Can you work these out from the model? Positions are in its coordinate system, mm. Face numbers are marked on the shaded views. A direction names the side the tool comes from. Give positions to 0.01 mm unless a question says otherwise; leave off trailing zeros. Write each loop counter-clockwise with the first axis right and the second up, starting at its lowest first coordinate (ties: lowest second). Pieces come first, ordered by that corner, then holes.
1. Thinking about a two-plate mould opening in Z: for the marked faces 1, 2, 3 and 4, which applies, pulls with the +Z half, pulls with the -Z half, needs draft (parallel to the pull), parting line crosses it, or undercut?
2. Suppose I cut it at B-B (y = -18). Please give me the cut outline in (x, z), and give its area (3 significant figures).
3. Suppose I cut it at A-A (x = 20). Please give me the cut outline in (y, z), and give its area (3 significant figures).
4. On a 3-axis mill with a long thin cutter (end or side, diameter ignored), from which of +Z, -Z, +X, -X, +Y, -Y can I reach the whole of each face in a straight line? I mean the marked faces 5, 6 and 7. Say none if no direction works.
5. Suppose I cut it at C-C (z = -28). Please give me the cut outline in (x, y).
6. If I drill on probe 1 along Y at (x, z) = (20, 3.85); probe 2 along X at (y, z) = (-18, 1.2); probe 3 along Y at (x, z) = (-37, -26.55), over which ranges is the centre line in solid material (lowest first)?
7. I'm going to push flat-ended pins straight in: pin 1 (1 mm diameter, centred on y = -2, z = -10.5, fed in from +X); pin 2 (10.5 mm diameter, centred on y = -10, z = -16, fed in from -X); pin 3 (3 mm diameter, centred on y = -10, z = -17, fed in from +X); pin 4 (4 mm diameter, centred on x = -21, y = -18.5, fed in from +Z). Where does each tip first touch, or does it pass through?
8. Suppose I cut it at D-D (y = 18). Please give me the cut outline in (x, z), and give its area (3 significant figures).
```python
from build123d import *

# Parameters (mm, degrees)
SKETCH1_W                      = 60
SKETCH1_H                      = 50
BOSS_EXTRUDE1_DEPTH            = 5
CUT_EXTRUDE1_DEPTH             = 40.37003937
CUT_EXTRUDE1_DEPTH_BACK        = 40.37003937
SKETCH5_R                      = 1.75
BOSS_EXTRUDE2_START            = -17
BOSS_EXTRUDE2_DEPTH            = 35
SKETCH6_W                      = 5.5
SKETCH6_H                      = 50
BOSS_EXTRUDE3_DEPTH            = 33
CUT_EXTRUDE2_DEPTH             = 71.32780389
CUT_EXTRUDE2_DEPTH_BACK        = 71.32780389
SKETCH7_R                      = 1.75
FILLET2_R                      = 3
FILLET3_R                      = 3
SKETCH8_R                      = 10.5
CUT_EXTRUDE3_DEPTH             = 28
FILLET4_R                      = 5
CBORE_FOR_M3_SHCS1_D           = 3.4
CBORE_FOR_M3_SHCS1_CBORE_D     = 6.5
CBORE_FOR_M3_SHCS1_CBORE_DEPTH = 3
SKETCH16_R                     = 1.7
CUT_EXTRUDE4_DEPTH             = 3
CHAMFER1_SIZE                  = 4


with BuildPart() as part:
    # Sketch1 → Boss-Extrude1 (new body)
    with BuildSketch(Plane.XY):
        Rectangle(SKETCH1_W, SKETCH1_H)
    extrude(amount=BOSS_EXTRUDE1_DEPTH)

    # Sketch5 → Cut-Extrude1 (cut, two sides: drawn at the far end of the back side and taken through both)
    with BuildSketch(Plane.XY.offset(5).offset(-CUT_EXTRUDE1_DEPTH_BACK)):
        with Locations((-20, 18)):
            Circle(SKETCH5_R)
        with Locations((20, 18)):
            Circle(SKETCH5_R)
        with Locations((20, -18)):
            Circle(SKETCH5_R)
        with Locations((-20, -18)):
            Circle(SKETCH5_R)
    extrude(amount=CUT_EXTRUDE1_DEPTH + CUT_EXTRUDE1_DEPTH_BACK, mode=Mode.SUBTRACT)

    # Sketch2 → Boss-Extrude2 (add)
    with BuildSketch(Plane(origin=(30, 0, 0), x_dir=(0, 0, -1), z_dir=(1, 0, 0)).offset(BOSS_EXTRUDE2_START)):
        Polygon((0, -25), (31, -25), (31, 25), (25.5, 25), (25.5, 8), (5.5, 8), (5.5, 25), (0, 25), align=None)
    extrude(amount=-BOSS_EXTRUDE2_DEPTH)

    # Sketch6 → Boss-Extrude3 (add)
    with BuildSketch(Plane.ZY.offset(22)):
        with Locations((-28.25, 0)):
            Rectangle(SKETCH6_W, SKETCH6_H)
    extrude(amount=BOSS_EXTRUDE3_DEPTH)

    # Sketch7 → Cut-Extrude2 (cut, two sides: drawn at the far end of the back side and taken through both)
    with BuildSketch(Plane(origin=(0, 0, -31), x_dir=(-1, 0, 0), z_dir=(0, 0, -1)).offset(-CUT_EXTRUDE2_DEPTH_BACK)):
        with Locations((37, 7.5)):
            Circle(SKETCH7_R)
        with Locations((44.5, 0)):
            Circle(SKETCH7_R)
        with Locations((37, -7.5)):
            Circle(SKETCH7_R)
        with Locations((29.5, 0)):
            Circle(SKETCH7_R)
    extrude(amount=CUT_EXTRUDE2_DEPTH + CUT_EXTRUDE2_DEPTH_BACK, mode=Mode.SUBTRACT)

    # Fillet2
    fillet2_edges = [part.edges().sort_by_distance(p)[0] for p in [
        (-22, 0, 0),
        (13, 0, 0),
    ]]
    fillet(fillet2_edges, radius=FILLET2_R)

    # Fillet3
    fillet3_edges = [part.edges().sort_by_distance(p)[0] for p in [
        (-4.5, 8, -5.5),
        (-4.5, 8, -25.5),
    ]]
    fillet(fillet3_edges, radius=FILLET3_R)

    # Sketch8 → Cut-Extrude3 (cut)
    with BuildSketch(Plane(origin=(0, 0, -31), x_dir=(-1, 0, 0), z_dir=(0, 0, -1))):
        with Locations((5, -10)):
            Circle(SKETCH8_R)
        with BuildLine():
            Line((-5.5, 0.5), (-5.5, -10))
            ThreePointArc((-5.5, -10), (-2.424621218, -2.575378813), (4.999999956, 0.5))
            Line((4.999999956, 0.5), (-5.5, 0.5))
        make_face()
        with BuildLine():
            ThreePointArc((4.999999956, 0.5), (12.424621187, -2.575378782), (15.5, -10))
            Line((15.5, -10), (15.5, 0.5))
            Line((15.5, 0.5), (4.999999956, 0.5))
        make_face()
        with BuildLine():
            Line((-5.5, -10), (-5.5, -20.5))
            Line((-5.5, -20.5), (5, -20.5))
            ThreePointArc((5, -20.5), (-2.424621202, -17.424621202), (-5.5, -10))
        make_face()
        with BuildLine():
            ThreePointArc((15.5, -10), (12.424621202, -17.424621202), (5, -20.5))
            Line((5, -20.5), (15.5, -20.5))
            Line((15.5, -20.5), (15.5, -10))
        make_face()
    extrude(amount=-CUT_EXTRUDE3_DEPTH, mode=Mode.SUBTRACT)

    # Fillet4
    fillet4_edges = [part.edges().sort_by_distance(p)[0] for p in [
        (-22, -7, -25.5),
    ]]
    fillet(fillet4_edges, radius=FILLET4_R)

    # CBORE for M3 SHCS1 (through all)
    with Locations(Plane.ZY.offset(22)):
        with Locations((-7.5, -10), (-16, -10)):
            CounterBoreHole(CBORE_FOR_M3_SHCS1_D / 2, CBORE_FOR_M3_SHCS1_CBORE_D / 2, CBORE_FOR_M3_SHCS1_CBORE_DEPTH)

    # Sketch16 → Cut-Extrude4 (cut)
    # profile 1 of 2: a face of its own
    with BuildSketch(Plane(origin=(13, 0, 0), x_dir=(0, 0, -1), z_dir=(1, 0, 0))):
        Polygon((5.875, -12.814582562), (9.125, -12.814582562), (10.75, -10), (9.125, -7.185417438), (5.875, -7.185417438), (4.25, -10), align=None)
        with Locations(Location((7.5, -10, 0), (0, 0, 180))):
            Circle(SKETCH16_R, mode=Mode.SUBTRACT)
    # profile 2 of 2: a face of its own
    with BuildSketch(Plane(origin=(13, 0, 0), x_dir=(0, 0, -1), z_dir=(1, 0, 0))):
        Polygon((14.375, -12.814582562), (17.625, -12.814582562), (19.25, -10), (17.625, -7.185417438), (14.375, -7.185417438), (12.75, -10), align=None)
        with Locations(Location((16, -10, 0), (0, 0, 180))):
            Circle(SKETCH16_R, mode=Mode.SUBTRACT)
    extrude(amount=-CUT_EXTRUDE4_DEPTH, mode=Mode.SUBTRACT)

    # Chamfer1
    chamfer1_edges = [part.edges().sort_by_distance(p)[0] for p in [
        (5.5, -10, -31),
        (-5, 0.5, -31),
        (-5, -20.5, -31),
        (-15.5, -10, -31),
    ]]
    chamfer(chamfer1_edges, length=CHAMFER1_SIZE)


solid = part.part
```
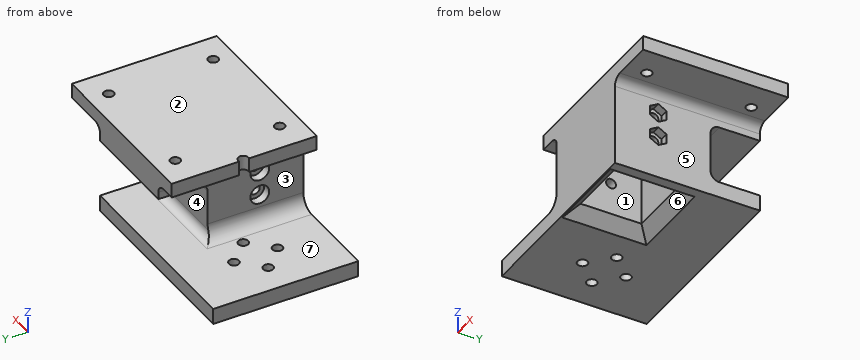
Checks:
1. face 1: needs draft
1. face 2: pulls with the +Z half
1. face 3: undercut
1. face 4: undercut
2. outline: (-55, -31) - (-19.5, -31) - (-15.5, -27) - (-15.5, -3) - (5.5, -3) - (5.5, -27) - (9.5, -31) - (13, -31) - (13, -3) arc R3 cw to (16, 0) - (18.25, 0) - (18.25, 5) - (-18.25, 5) - (-18.25, 0) - (-21.75, 0) - (-21.75, 5) - (-30, 5) - (-30, 0) - (-25, 0) arc R3 cw to (-22, -3) - (-22, -20.5) arc R5 cw to (-27, -25.5) - (-55, -25.5) - close; (21.75, 0) - (30, 0) - (30, 5) - (21.75, 5) - close
2. area: 937 mm2
3. outline: (-25, 0) - (-19.75, 0) - (-19.75, 5) - (-25, 5) - close; (-16.25, 0) - (16.25, 0) - (16.25, 5) - (-16.25, 5) - close; (19.75, 0) - (25, 0) - (25, 5) - (19.75, 5) - close
3. area: 215 mm2
4. face 5: -Z, +X, +Y, -Y
4. face 6: -Z
4. face 7: -X, +Y
5. outline: (-55, -25) - (13, -25) - (13, 25) - (-55, 25) - close; hole circle Ø3.5 at (-44.5, 0); hole circle Ø3.5 at (-37, -7.5); hole circle Ø3.5 at (-37, 7.5); hole circle Ø3.5 at (-29.5, 0); hole (-16.5, -21.5) - (6.5, -21.5) - (6.5, 1.5) - (-16.5, 1.5) - close
6. probe 1: y = -25 to -19.75, -16.25 to 16.25, 19.75 to 25
6. probe 2: x = -30 to -21.75, -18.25 to 18.25, 21.75 to 30
6. probe 3: y = -25 to -9.25, -5.75 to 5.75, 9.25 to 25
7. pin 1: stops at x = 13
7. pin 2: stops at x = -22.06
7. pin 3: stops at x = 10
7. pin 4: stops at z = 5
8. outline: (-55, -31) - (13, -31) - (13, -25.5) - (-55, -25.5) - close; (-30, 0) - (-25, 0) arc R3 cw to (-22, -3) - (-22, -5.5) - (13, -5.5) - (13, -3) arc R3 cw to (16, 0) - (18.25, 0) - (18.25, 5) - (-18.25, 5) - (-18.25, 0) - (-21.75, 0) - (-21.75, 5) - (-30, 5) - close; (21.75, 0) - (30, 0) - (30, 5) - (21.75, 5) - close
8. area: 835 mm2
